from build123d import *

# Parameters (mm, degrees)
F0_R     = 117.18925
F0_R_2   = 98.46945
F1_DEPTH = 14.1224
F2_R     = 98.4885
F2_R_2   = 93.98
F3_DEPTH = 1524
F4_R     = 117.18925
F4_R_2   = 98.46945
F5_DEPTH = 25.4
F6_R     = 4.96062
F7_DEPTH = 1524.001


with BuildPart() as f1:
    # F0 (on Top) → F1 (new body)
    with BuildSketch(Plane.XY):
        Circle(F0_R)
        Circle(F0_R_2, mode=Mode.SUBTRACT)
    extrude(amount=F1_DEPTH)

    # F2 (on face) → F3 (join)
    with BuildSketch(Plane(origin=(0, 0, 0), x_dir=(1, 0, 0), z_dir=(0, 0, -1))):
        Circle(F2_R)
        Circle(F2_R_2, mode=Mode.SUBTRACT)
    extrude(amount=-F3_DEPTH)

    # F4 (on face) → F5 (join)
    with BuildSketch(Plane.XY.offset(1524)):
        Circle(F4_R)
        Circle(F4_R_2, mode=Mode.SUBTRACT)
    extrude(amount=-F5_DEPTH)

    # F6 (on face) → F7 (cut, through all)
    with BuildSketch(Plane.XY.offset(1524)):
        with Locations((0, -108.24972)):
            Circle(F6_R)
        with Locations((54.12486, -93.747007)):
            Circle(F6_R)
        with Locations((93.747007, -54.12486)):
            Circle(F6_R)
        with Locations((108.24972, 0)):
            Circle(F6_R)
        with Locations((93.747007, 54.12486)):
            Circle(F6_R)
        with Locations((54.12486, 93.747007)):
            Circle(F6_R)
        with Locations((0, 108.24972)):
            Circle(F6_R)
        with Locations((-54.12486, 93.747007)):
            Circle(F6_R)
        with Locations((-93.747007, 54.12486)):
            Circle(F6_R)
        with Locations((-108.24972, 0)):
            Circle(F6_R)
        with Locations((-93.747007, -54.12486)):
            Circle(F6_R)
        with Locations((-54.12486, -93.747007)):
            Circle(F6_R)
    extrude(amount=-F7_DEPTH, mode=Mode.SUBTRACT)


solid = f1.part
Build history of the part. All positions in model axes, mm. A direction names the side the tool comes from. Give positions to 0.01 mm unless a question says otherwise; leave off trailing zeros. Write each loop counter-clockwise with the first axis right and the second up, starting at its lowest first coordinate (ties: lowest second). Pieces come first, ordered by that corner, then holes. Notation, with made-up numbers: (45, -25.75) - (76, -25.75) arc R16 ccw to (76, 3.25) - close; hole circle Ø4 at (15.25, 67.5). An arc over 180 degrees is marked (long way). Use one line per item in the form item = value. Start each with the question number.
1. Probe line 1 (Z direction, x = 81.5, y = -70); line 2 (X direction, y = -1, z = 367); line 3 (Y direction, x = -23, z = 1006.5). List the from-to ranges inside material, lowest first. Write a range as [from, to].
2. Two-plate mould, pull along Y, no slides. Class faces 3 (the face through (-92.997, -71.308, 1511.478)), 4 (the face through (-20.373, 91.745, 751.332)), 5 (the face through (-53, 79, 0)): released by +Y, released by -Y, zero draft, split by the parting line, or undercut.
3. Drop flat-ended pins along their axis: pin 1 Ø6 at (x, y) = (93.75, 54.12) entering from +Z; pin 2 Ø12 at (x, z) = (23.5, 503) entering from +Y; pin 3 Ø10 at (y, z) = (28, 669) entering from +X; pin 4 Ø12 at (y, z) = (-56, 291) entering from +X. Give the stop position or say it passes through.
4. Band-saw the part on B-B on z = 760.5. Write the cut outline in (x, y).
5. Band-saw the part on A-A on y = 24. Write the cut outline in (x, z).
6. 3-axis set-ups, long thin cutter, end or side, ignore diameter. For faces 1 (the face through (93.94, -29.58, 745.97)), 2 (the face through (-53, 79, 1524)): which of +Z, -Z, +X, -X, +Y, -Y reach the whole face in a straight line?
Conclusion:
q1.line_1 = [0, 14.12], [1498.6, 1524]
q1.line_2 = [-98.48, -93.97], [93.97, 98.48]
q1.line_3 = [-95.77, -91.12], [91.12, 95.77]
q2.face_3 = split by the parting line
q2.face_4 = undercut
q2.face_5 = zero draft
q3.pin_1 = through
q3.pin_2 = 96.92
q3.pin_3 = 95.77
q3.pin_4 = 84.85
q4.outline = circle Ø196.98 at (0, 0); hole circle Ø187.96 at (0, 0)
q5.outline = (-114.71, 0) - (-90.86, 0) - (-90.86, 1524) - (-114.71, 1524) - (-114.71, 1498.6) - (-95.52, 1498.6) - (-95.52, 14.12) - (-114.71, 14.12) - close; (90.86, 0) - (114.71, 0) - (114.71, 14.12) - (95.52, 14.12) - (95.52, 1498.6) - (114.71, 1498.6) - (114.71, 1524) - (90.86, 1524) - close
q6.face_1 = none
q6.face_2 = +Z, +X, -X, +Y, -Y
